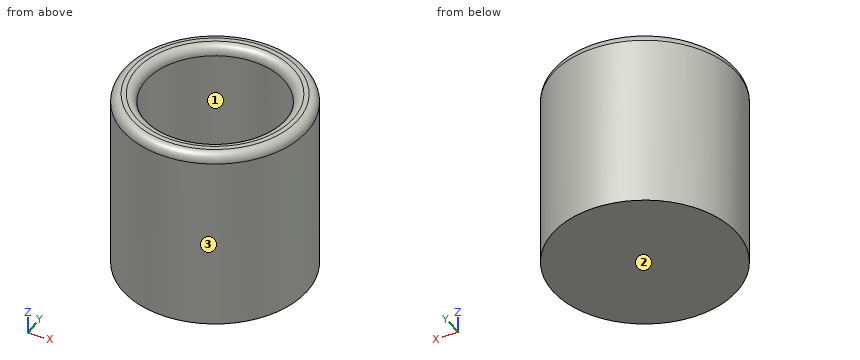
from build123d import *

# Parameters (mm, degrees)
F0_R     = 152.4
F1_DEPTH = 304.8
F2_R     = 114.3
F3_DEPTH = 228.6
F4_R     = 15.24


with BuildPart() as f1:
    # F0 (on Top) → F1 (new body)
    with BuildSketch(Plane.XY):
        with Locations((-36.681142, 40.239949)):
            Circle(F0_R)
    extrude(amount=F1_DEPTH)

    # F2 (on face) → F3 (cut)
    with BuildSketch(Plane.XY.offset(304.8)):
        with Locations((-36.681142, 40.239949)):
            Circle(F2_R)
    extrude(amount=-F3_DEPTH, mode=Mode.SUBTRACT)

    # F4
    f4_edges = [f1.edges().sort_by_distance(p)[0] for p in [
        (-150.981142, 40.239949, 304.8),
        (-189.081142, 40.239949, 304.8),
    ]]
    fillet(f4_edges, radius=F4_R)


solid = f1.part
Can you work these out from the model? Positions are in its coordinate system, mm. Face numbers are marked on the shaded views. Round coordinates to 2 decimals unless told otherwise and drop trailing zeros. Write each loop counter-clockwise with the first axis right and the second up, starting at its lowest first coordinate (ties: lowest second). Pieces come first, ordered by that corner, then holes. Notation, with made-up numbers: M 59.5,-3 L 105.5,-3 A26 ccw 105.5,30 Z; hole C -10,9 d9. An arc over 180 degrees is marked long. Use CSV: the item, a comma, the result in double quotes.
(1) I'm going to push flat-ended pins straight in: pin 1 (3 mm diameter, centred on x = 42.5, z = 209, fed in from +Y); pin 2 (6 mm diameter, centred on x = 44, z = 207.5, fed in from -Y); pin 3 (1 mm diameter, centred on x = -125.5, z = 203.5, fed in from -Y). Where does each tip first touch, or does it pass through?
Check values:
pin 1,"y = 171.36"
pin 2,"y = -90.88"
pin 3,"y = -83.96"
(2) I need wall thicknesses on line 1 along X through (y, z) = (39.5, 272); line 2 along Y through (x, z) = (-76, 292); line 3 along Z through (x, y) = (-91, 57). Which ranges of each line are inside material? Lowest first, please.
Check values:
line 1,"-189.08 to -150.98, 77.62 to 115.72"
line 2,"-106.8 to -67.29, 147.77 to 187.28"
line 3,"0 to 76.2"
(3) Imagine slicing it at A-A (z = 174). Write out the boundary of the cut face in (x, y), plus the area to 3 significant figures.
Check values:
outline,"C -36.68,40.24 d304.8; hole C -36.68,40.24 d228.6"
area,"31,900 mm^2"
(4) We'd pull the mould along X, two halves only. Please class the marked faces 1, 2 and 3: +X half, -X half, draft (parallel to the pull), parting line (faces both ways), or undercut.
Check values:
face 1,"undercut"
face 2,"draft"
face 3,"parting line"
